from build123d import *

# Parameters (mm, degrees)
BOSS_EXTRUDE1_DEPTH     = 16
BOSS_EXTRUDE2_START     = -16
BOSS_EXTRUDE2_DEPTH     = 16
FILLET1_R               = 10
SKETCH3_R               = 9
BOSS_EXTRUDE3_DEPTH     = 6
CUT_EXTRUDE1_DEPTH      = 47.217444076
CUT_EXTRUDE1_DEPTH_BACK = 47.217444076
SKETCH5_R               = 1.65
SKETCH10_R              = 2.85
CUT_EXTRUDE4_DEPTH      = 57.367261237


with BuildPart() as part:
    # Sketch1 → Boss-Extrude1 (new body)
    with BuildSketch(Plane(origin=(0, 0, 0), x_dir=(1, 0, 0), z_dir=(0, 1, 0))):
        with BuildLine():
            ThreePointArc((-22.806656603, 2.975972883), (-23, 0), (-22.806656603, -2.975972883))
            ThreePointArc((-22.806656603, -2.975972883), (-12.124355653, -7), (-13.980596419, -18.263157552))
            ThreePointArc((-13.980596419, -18.263157552), (-11.5, -19.918584287), (-8.826060184, -21.239130435))
            ThreePointArc((-8.826060184, -21.239130435), (0, -14), (8.826060184, -21.239130435))
            ThreePointArc((8.826060184, -21.239130435), (11.5, -19.918584287), (13.980596419, -18.263157552))
            ThreePointArc((13.980596419, -18.263157552), (12.124355653, -7), (22.806656603, -2.975972883))
            ThreePointArc((22.806656603, -2.975972883), (23, 0), (22.806656603, 2.975972883))
            ThreePointArc((22.806656603, 2.975972883), (12.124355653, 7), (13.980596419, 18.263157552))
            ThreePointArc((13.980596419, 18.263157552), (11.5, 19.918584287), (8.826060184, 21.239130435))
            ThreePointArc((8.826060184, 21.239130435), (0, 14), (-8.826060184, 21.239130435))
            ThreePointArc((-8.826060184, 21.239130435), (-11.5, 19.918584287), (-13.980596419, 18.263157552))
            ThreePointArc((-13.980596419, 18.263157552), (-12.124355653, 7), (-22.806656603, 2.975972883))
        make_face()
    extrude(amount=BOSS_EXTRUDE1_DEPTH)

    # Sketch2 → Boss-Extrude2 (add)
    with BuildSketch(Plane(origin=(0, 16, 0), x_dir=(1, 0, 0), z_dir=(0, 1, 0)).offset(BOSS_EXTRUDE2_START)):
        with BuildLine():
            ThreePointArc((-13.980596419, 18.263157552), (-16.774955839, 19.933125173), (-19.980596419, 20.499786358))
            ThreePointArc((-19.980596419, 20.499786358), (-21.238909345, 23.025125967), (-19.040914816, 24.794168535))
            ThreePointArc((-19.040914816, 24.794168535), (-13.4912909, 24.287233332), (-8.826060184, 21.239130435))
            ThreePointArc((-8.826060184, 21.239130435), (-11.5, 19.918584287), (-13.980596419, 18.263157552))
        make_face()
        with BuildLine():
            ThreePointArc((13.980596419, 18.263157552), (11.5, 19.918584287), (8.826060184, 21.239130435))
            ThreePointArc((8.826060184, 21.239130435), (8.875114857, 24.494100491), (7.763037549, 27.553597261))
            ThreePointArc((7.763037549, 27.553597261), (9.32088934, 29.905998025), (11.951922409, 28.88700021))
            ThreePointArc((11.951922409, 28.88700021), (14.287715603, 23.827417316), (13.980596419, 18.263157552))
        make_face()
        with BuildLine():
            ThreePointArc((22.806656603, -2.975972883), (23, 0), (22.806656603, 2.975972883))
            ThreePointArc((22.806656603, 2.975972883), (25.650070696, 4.560975318), (27.743633968, 7.053810902))
            ThreePointArc((27.743633968, 7.053810902), (30.559798685, 6.880872058), (30.992837225, 4.092831674))
            ThreePointArc((30.992837225, 4.092831674), (27.779006503, -0.459816017), (22.806656603, -2.975972883))
        make_face()
        with BuildLine():
            ThreePointArc((8.826060184, -21.239130435), (11.5, -19.918584287), (13.980596419, -18.263157552))
            ThreePointArc((13.980596419, -18.263157552), (16.774955839, -19.933125173), (19.980596419, -20.499786358))
            ThreePointArc((19.980596419, -20.499786358), (21.238909345, -23.025125967), (19.040914816, -24.794168535))
            ThreePointArc((19.040914816, -24.794168535), (13.4912909, -24.287233332), (8.826060184, -21.239130435))
        make_face()
        with BuildLine():
            ThreePointArc((-13.980596419, -18.263157552), (-11.5, -19.918584287), (-8.826060184, -21.239130435))
            ThreePointArc((-8.826060184, -21.239130435), (-8.875114857, -24.494100491), (-7.763037549, -27.553597261))
            ThreePointArc((-7.763037549, -27.553597261), (-9.32088934, -29.905998025), (-11.951922409, -28.88700021))
            ThreePointArc((-11.951922409, -28.88700021), (-14.287715603, -23.827417316), (-13.980596419, -18.263157552))
        make_face()
        with BuildLine():
            ThreePointArc((-22.806656603, 2.975972883), (-23, 0), (-22.806656603, -2.975972883))
            ThreePointArc((-22.806656603, -2.975972883), (-25.650070696, -4.560975318), (-27.743633968, -7.053810902))
            ThreePointArc((-27.743633968, -7.053810902), (-30.559798685, -6.880872058), (-30.992837225, -4.092831674))
            ThreePointArc((-30.992837225, -4.092831674), (-27.779006503, 0.459816017), (-22.806656603, 2.975972883))
        make_face()
    extrude(amount=BOSS_EXTRUDE2_DEPTH)

    # Fillet1
    fillet1_edges = [part.edges().sort_by_distance(p)[0] for p in [
        (13.980596419, 8, -18.263157552),
        (22.806656603, 8, 2.975972883),
        (8.826060184, 8, 21.239130435),
        (-13.980596419, 8, 18.263157552),
        (-22.806656603, 8, -2.975972883),
        (-8.826060184, 8, -21.239130435),
    ]]
    fillet(fillet1_edges, radius=FILLET1_R)

    # Sketch3 → Boss-Extrude3 (add)
    with BuildSketch(Plane.XZ):
        with Locations(Location((0, 0, 0), (0, 0, 90))):
            Circle(SKETCH3_R)
    extrude(amount=BOSS_EXTRUDE3_DEPTH)

    # Sketch5 → Cut-Extrude1 (cut, two sides: drawn at the far end of the back side and taken through both)
    with BuildSketch(Plane.XY.offset(-CUT_EXTRUDE1_DEPTH_BACK)):
        with Locations((0, -2.436)):
            Circle(SKETCH5_R)
    extrude(amount=CUT_EXTRUDE1_DEPTH + CUT_EXTRUDE1_DEPTH_BACK, mode=Mode.SUBTRACT)

    # Sketch6 → Revolve1 (revolve)
    with BuildSketch(Plane.XY, mode=Mode.PRIVATE) as revolve1_sk:
        Polygon((-0.426503876, 16), (-0.426503876, 26), (11.573496124, 16), align=None)
    revolve(revolve1_sk.sketch.rotate(Axis((-0.426503876, 16, 0), (0, 1, 0)), 90), axis=Axis((-0.426503876, 16, 0), (0, 1, 0)))

    # Sketch10 → Cut-Extrude4 (cut, through all)
    with BuildSketch(Plane.XY.offset(9)):
        with Locations((0, -2.436)):
            Circle(SKETCH10_R)
    cut_extrude4 = extrude(amount=CUT_EXTRUDE4_DEPTH, mode=Mode.SUBTRACT)

    # Mirror1: Cut-Extrude4 across plane
    add(cut_extrude4.mirror(Plane.XY), mode=Mode.SUBTRACT)


solid = part.part
Work out the finished part from the listing and answer in its coordinate system (mm). A direction names the side the tool comes from. Give positions to 0.01 mm unless a question says otherwise; leave off trailing zeros. Write each loop counter-clockwise with the first axis right and the second up, starting at its lowest first coordinate (ties: lowest second). Pieces come first, ordered by that corner, then holes. Notation, with made-up numbers: (27.25, 66) - (42.25, 66) arc R23 ccw to (42.25, 93) - close; hole circle Ø5 at (78, -38). An arc over 180 degrees is marked (long way). One line per item, written item: value. Start each with the question number.
1. Consider probe 1 along Z at (x, y) = (12, 3); probe 2 along X at (y, z) = (4, 11); probe 3 along Y at (x, z) = (12.5, -26). Determine where each line is inside the solid, lowest interval first.
2. For faces 1 (the cylindrical face through (0.022, 0.414, -11.525)), 2 (the flat face through (-12, 0, -2)), 3 (the flat face through (12, 0, -1)), 4 (the cylindrical face through (-2.703, -2.958, 8.584)), 5 (the flat face through (12, 16, 0)), determine the directions among +Z, -Z, +X, -X, +Y, -Y from which every point of the face is accessible in a straight line to the end or side of a thin tool.
3. For a pull along Y with two mould halves and no side action, classify faces 6 (the conical face through (1.61, 24.26, 0.45)), 7 (the cylindrical face through (-0.358, -4.047, -0.126)), 8 (the cylindrical face through (-17.862, 7.888, -24.914)), 9 (the flat face through (0, -6, 0)) as +Y half, -Y half, draft (parallel to the pull), parting line (faces both ways), or undercut.
4. Find section A-A (z = -13). Write down the section's boundary in (x, y), then the cut area to 3 significant figures.
5. Given pin 1 (8 mm diameter, centred on x = 22, y = 15.5, fed in from +Z); pin 2 (3 mm diameter, centred on y = 15.5, z = 1, fed in from +X); pin 3 (8 mm diameter, centred on x = 19.5, z = 22, fed in from +Y), each flat-ended and moving along its own axis, determine where each tip first touches the part or whether it passes through.
Geometry results:
1. probe 1: -28.83 to -15.78, -7.22 to 7.22, 15.78 to 23.47
1. probe 2: -10.93 to 10.93
1. probe 3: 0 to 16
2. face 1: -Z, -Y
2. face 2: -X, -Y
2. face 3: +X, -Y
2. face 4: -Y
2. face 5: +Y
3. face 6: +Y half
3. face 7: undercut
3. face 8: draft
3. face 9: -Y half
4. outline: (-11.04, 0) - (-1.48, 0) arc R2.85 cw to (1.48, 0) - (11.04, 0) - (11.04, 16) - (-11.04, 16) - close
4. area: 353 mm2
5. pin 1: z = 24.91
5. pin 2: x = 28.73
5. pin 3: y = 16
